Autodesk Inventor part; units mm, degrees
ref_plane "YZ Plane" through (0, 0, 0) normal (1, 0, 0) x (0, 1, 0)
ref_plane "XZ Plane" through (0, 0, 0) normal (0, 1, 0) x (-1, 0, 0)
ref_plane "XY Plane" through (0, 0, 0) normal (0, 0, 1) x (1, 0, 0)
sketch "Sketch1" plane through (0, 0, 0) normal (0, 1, 0) x (-1, 0, 0)
  circle A0 centre (0, 0) radius 4.75
  circle A1 centre (0, 0) radius 6.25
  dimension "d0" = 9.5
  dimension "d1" = 1.5
extrude "Extrusion1" add sketch "Sketch1" along normal blind 100
sketch "Sketch2" plane through (0, 0, 0) normal (0, -1, 0) x (1, 0, 0)
  line L0 (-6.25, -0.2) -> (6.25, -0.2)
  line L1 (6.25, -0.2) -> (6.25, 0.2)
  line L2 (6.25, 0.2) -> (-6.25, 0.2)
  line L3 (-6.25, 0.2) -> (-6.25, -0.2)
  line L4 (-0.2, 6.25) -> (-0.2, -6.25)
  line L5 (0.2, -6.25) -> (0.2, 6.25)
  line L6 (-0.2, -6.25) -> (0.2, -6.25)
  line L7 (0.2, 6.25) -> (-0.2, 6.25)
  line L8 (-6.25, -0.2) -> (6.25, -0.2)
  line L9 (6.25, 0.2) -> (-6.25, 0.2)
  line L10 (6.25, -0.2) -> (6.25, 0.2)
  line L11 (-6.25, 0.2) -> (-6.25, -0.2)
  line L12 (0.2, -6.25) -> (0.2, 6.25)
  line L13 (-0.2, 6.25) -> (-0.2, -6.25)
  line L14 (0.2, 6.25) -> (-0.2, 6.25)
  line L15 (-0.2, -6.25) -> (0.2, -6.25)
  point P0 (0, 0)
  point P1 (0.2, -0.2)
  point P2 (0.2, 0.2)
  point P3 (-0.2, 0.2)
  point P4 (-0.2, -0.2)
  dimension "d4" = 12.5
  dimension "d5" = 6.25
  dimension "d6" = 0.4
  dimension "d7" = 0.2
  dimension "d10" = 360
extrude "Extrusion2" cut sketch "Sketch2" against normal blind 12
fillet "Fillet1" radius 1.2 4 edges at (-3.3588, 0, -3.3588) (3.3588, 0, -3.3588) (3.3588, 0, 3.3588) (-3.3588, 0, 3.3588)
properties part number "Turret_extend"
Input: part model. Units: mm. Frame: model coordinates. Give positions to 0.01 mm unless a question says otherwise; leave off trailing zeros. Order: outer loops, then holes, each group sorted by start corner. A loop starts at its lowest first (then second) coordinate and runs counter-clockwise, first axis right, second up. Notation, with made-up numbers: M 15,37.5 L 60,37.5 A33 ccw 60,67.5 Z; hole C 67.5,13.5 d1. An arc over 180 degrees is marked long. Return JSON: item names as keys, results as strings.
Item 1: Pull-direction query (X, two-part tool) for faces 1 (the cylindrical face through (-5.96, 49.3, -1.88)), 2 (the flat face through (1, 100, 5)), 3 (the cylindrical face through (-2.192, 49.908, 4.214)); classes: +X half, -X half, draft (parallel to the pull), parting line (faces both ways), or undercut.
Solutions:
{"face 1": "parting line", "face 2": "draft", "face 3": "undercut"}
Item 2: Ray query, probe 1 along X at (y, z) = (24.5, 0); probe 2 along Y at (x, z) = (-1, 5.75). Return the intervals inside material, ascending.
Solutions:
{"probe 1": "-6.25 to -4.75, 4.75 to 6.25", "probe 2": "0.01 to 100"}
Item 3: Cut plane A-A (y = 41.5). Return loops of the section in (x, z), then the cut area to 3 significant figures.
Solutions:
{"outline": "C 0,0 d12.5; hole C 0,0 d9.5", "area": "51.8 mm^2"}
Item 4: First-contact query: P1, Ø0.8, axis at y = 8, z = 5.5, coming from the +X side; P2, Ø1.2, axis at y = 5.5, z = -5.5, coming from the -X side; P3, Ø0.8, axis at y = 8, z = 5, coming from the -X side. Flat tips, straight axial feed; report the tip coordinate or a pass-through.
Solutions:
{"P1": "x = 3.61", "P2": "x = -3.88", "P3": "x = -4.23"}
